from build123d import *

# Parameters (mm, degrees)
SKETCH1_W                = 25
SKETCH1_H                = 250
BOSS_EXTRUDE1_DEPTH      = 20
SKETCH2_W                = 120
SKETCH2_H                = 4
BOSS_EXTRUDE2_DEPTH      = 20
CUT_EXTRUDE1_DEPTH       = 20
LPATTERN1_COUNT          = 5
LPATTERN1_PITCH          = 30
LPATTERN1_COL_COUNT      = 4
LPATTERN1_COL_PITCH      = 30
FILLET1_R                = 5
BOSS_EXTRUDE4_DEPTH      = 5
BOSS_EXTRUDE4_DEPTH_BACK = 5
FILLET2_R                = 5
CHAMFER1_SIZE            = 10


with BuildPart() as part:
    # Sketch1 → Boss-Extrude1 (new body)
    with BuildSketch(Plane.XY):
        Rectangle(SKETCH1_W, SKETCH1_H)
    extrude(amount=BOSS_EXTRUDE1_DEPTH)

    # Sketch2 → Boss-Extrude2 (add)
    with BuildSketch(Plane.XY):
        with Locations((0, 127)):
            Rectangle(SKETCH2_W, SKETCH2_H)
    extrude(amount=BOSS_EXTRUDE2_DEPTH)

    # Sketch5 → Cut-Extrude1 (cut)
    with BuildSketch(Plane(origin=(0, 0, 0), x_dir=(1, 0, 0), z_dir=(0, 1, 0))):
        with BuildLine():
            Line((1.199542867, -0.052363953), (1.199542867, 0))
            Line((1.199542867, 0), (12.5, 0))
            Line((12.5, 0), (12.5, -8))
            ThreePointArc((12.5, -8), (7.91900236, -2.505881075), (1.199542867, -0.052363953))
        make_face()
        with BuildLine():
            Line((-1.199542867, -0.052363953), (-1.199542867, 0))
            Line((-1.199542867, 0), (-12.5, 0))
            Line((-12.5, 0), (-12.5, -8))
            ThreePointArc((-12.5, -8), (-7.91900236, -2.505881075), (-1.199542867, -0.052363953))
        make_face()
    cut_extrude1 = extrude(amount=-CUT_EXTRUDE1_DEPTH, mode=Mode.SUBTRACT)

    # LPattern1: Cut-Extrude1 ×5
    with Locations(*[(0, -i * LPATTERN1_PITCH, 0) for i in range(1, LPATTERN1_COUNT)]):
        add(cut_extrude1, mode=Mode.SUBTRACT)

    # LPattern1 col: Cut-Extrude1 ×4
    with Locations(*[(0, i * LPATTERN1_COL_PITCH, 0) for i in range(1, LPATTERN1_COL_COUNT)]):
        add(cut_extrude1, mode=Mode.SUBTRACT)

    # Fillet1
    fillet1_edges = [part.edges().sort_by_distance(p)[0] for p in [
        (12.5, 5, 0),
        (-12.5, -25, 0),
        (-12.5, 65, 0),
        (-12.5, 35, 0),
        (-12.5, 5, 0),
        (12.5, 35, 0),
        (12.5, 65, 0),
        (12.5, -115, 0),
        (12.5, -85, 0),
        (12.5, -55, 0),
        (12.5, -25, 0),
        (-12.5, -55, 0),
        (-12.5, -85, 0),
        (-12.5, -115, 0),
    ]]
    fillet(fillet1_edges, radius=FILLET1_R)

    # Sketch6 → Boss-Extrude4 (add, two sides: drawn at the far end of the back side and taken through both)
    with BuildSketch(Plane(origin=(0, 0, 0), x_dir=(0, 0, -1), z_dir=(1, 0, 0)).offset(-BOSS_EXTRUDE4_DEPTH_BACK)):
        Polygon((-20, 49), (-80, 129), (-98.75, 129), (-20, 24), align=None)
    extrude(amount=BOSS_EXTRUDE4_DEPTH + BOSS_EXTRUDE4_DEPTH_BACK)

    # Fillet2
    fillet2_edges = [part.edges().sort_by_distance(p)[0] for p in [
        (-12.5, 0, 20),
        (12.5, 0, 20),
    ]]
    fillet(fillet2_edges, radius=FILLET2_R)

    # Chamfer1
    # the kernel refuses this chamfer: 10 mm, written as the material it adds along each edge
    with BuildSketch(Plane(origin=(12.5, 125, 0), x_dir=(-0.027495876610586147, -0.9996219169112968, 0), z_dir=(0, 0, 1))) as chamfer1_piece_1:
        Polygon((CHAMFER1_SIZE * 0.999621916911, CHAMFER1_SIZE * 0.0274958766106), (-CHAMFER1_SIZE * 0.0274958766106, CHAMFER1_SIZE * 0.999621916911), (0, 0), align=None)
    extrude(amount=15)
    with BuildSketch(Plane(origin=(-12.5, 125, 0), x_dir=(0.02749587661058649, -0.9996219169112968, 0), z_dir=(0, 0, 1))) as chamfer1_piece_2:
        Polygon((CHAMFER1_SIZE * 0.999621916911, -CHAMFER1_SIZE * 0.0274958766106), (-CHAMFER1_SIZE * 0.0274958766106, -CHAMFER1_SIZE * 0.999621916911), (0, 0), align=None)
    extrude(amount=15)
    with BuildSketch(Plane(origin=(7.5, 125, 15), x_dir=(1, 0, 0), z_dir=(0, 0, -1))) as chamfer1_piece_3_section:
        Polygon((5, CHAMFER1_SIZE), (5 + CHAMFER1_SIZE, 0), (5, 0), align=None)
    chamfer1_piece_3 = revolve(axis=Axis((7.5, 125, 15), (0, -1, 0)), revolution_arc=359.64, mode=Mode.PRIVATE)
    chamfer1_piece_3 = split(chamfer1_piece_3, bisect_by=Plane(origin=(11.362208606, 120.302173253, 20), z_dir=(0, 0, -1)), keep=Keep.TOP, mode=Mode.PRIVATE)
    add(chamfer1_piece_3)
    with BuildSketch(Plane(origin=(-7.5, 125, 15), x_dir=(-1, 0, 0), z_dir=(0, 0, -1))) as chamfer1_piece_4_section:
        Polygon((5 + CHAMFER1_SIZE, 0), (5, -CHAMFER1_SIZE), (5, 0), align=None)
    chamfer1_piece_4 = revolve(axis=Axis((-7.5, 125, 15), (0, 1, 0)), revolution_arc=359.64, mode=Mode.PRIVATE)
    chamfer1_piece_4 = split(chamfer1_piece_4, bisect_by=Plane(origin=(-15.762682171, 121.86864034, 20), z_dir=(0, 0, -1)), keep=Keep.TOP, mode=Mode.PRIVATE)
    add(chamfer1_piece_4)


solid = part.part
Check sheet for the modelled part. Datum: model origin and axes. Units: mm. A direction names the side the tool comes from. Give positions to 0.01 mm unless a question says otherwise; leave off trailing zeros. Write each loop counter-clockwise with the first axis right and the second up, starting at its lowest first coordinate (ties: lowest second). Pieces come first, ordered by that corner, then holes. Notation, with made-up numbers: (60, 48) -> (101, 48) arc R34 ccw to (101, 87) -> close; hole circle Ø8 at (85, -27). An arc over 180 degrees is marked (long way). One line per item, written item: value. Start each with the question number.
Item 1: Gauge pin test, flat ends, axial feed: pin 1 (5 mm diameter, centred on y = 53.5, z = 32.5, fed in from +X); pin 2 (8 mm diameter, centred on y = 94.5, z = 21.5, fed in from +X); pin 3 (8 mm diameter, centred on x = 19, z = 14.5, fed in from -Y). Record the tip position at first contact, or that the pin passes through.
Item 2: Material ranges on probe 1 along X at (y, z) = (-112, 11); probe 2 along Y at (x, z) = (-26, 10); probe 3 along Z at (x, y) = (6.5, -54), recorded low to high. Write a range as from..to.
Item 3: Section check C-C on y = -41.5. Record the cut outline in (x, z).
Item 4: Section check B-B on z = 12. Record the cut outline in (x, y), then the cut area to 3 significant figures.
Item 5: Draft check along Y on faces 1 (the cylindrical face through (-11, -54.93, 1.43)), 2 (the flat face through (9, -120, 2)), 3 (the cylindrical face through (8.002, 80.14, 2.564)). Enter one of: +Y half, -Y half, draft (parallel to the pull), parting line (faces both ways), or undercut.
Item 6: Section check D-D on x = -34. Record the cut outline in (y, z), then the cut area to 3 significant figures.
Item 7: Section check A-A on y = 104. Record the cut outline in (x, z).
Item 8: Tool access check on faces 4 (the cylindrical face through (11, -54.93, 1.43)), 5 (the cylindrical face through (-11, -114.93, 1.43)), 6 (the cylindrical face through (8.002, 50.14, 2.564)), 7 (the cylindrical face through (-8.002, -9.86, 2.564)). Record the directions out of +Z, -Z, +X, -X, +Y, -Y that give a thin tool (end or side, any length) a straight path to the whole face; none if there is none.
Results list:
1. pin 1: x = 5
1. pin 2: x = 11.83
1. pin 3: y = 117.5
2. probe 1: -12.5..12.5
2. probe 2: 125..129
2. probe 3: 0..20
3. outline: (-12.5, 8) arc R13.77 ccw to (-1.2, 0.05) -> (-1.2, 0) -> (1.2, 0) -> (1.2, 0.05) arc R13.77 ccw to (12.5, 8) -> (12.5, 15) arc R5 ccw to (7.5, 20) -> (-7.5, 20) arc R5 ccw to (-12.5, 15) -> close
4. outline: (-60, 125) -> (-22.5, 125) -> (-12.5, 115) -> (-12.5, -125) -> (12.5, -125) -> (12.5, 115) -> (22.5, 125) -> (60, 125) -> (60, 129) -> (-60, 129) -> close
4. area: 6,830 mm²
5. face 1: draft
5. face 2: -Y half
5. face 3: undercut
6. outline: (125, 0) -> (129, 0) -> (129, 20) -> (125, 20) -> close
6. area: 80.0 mm²
7. outline: (-12.5, 0) -> (12.5, 0) -> (12.5, 15) arc R5 ccw to (7.5, 20) -> (-7.5, 20) arc R5 ccw to (-12.5, 15) -> close; (-5, 61.25) -> (5, 61.25) -> (5, 80) -> (-5, 80) -> close
8. face 4: -Z, +X, -Y
8. face 5: -Z, -X, -Y
8. face 6: -Z, +X
8. face 7: -Z, -X
